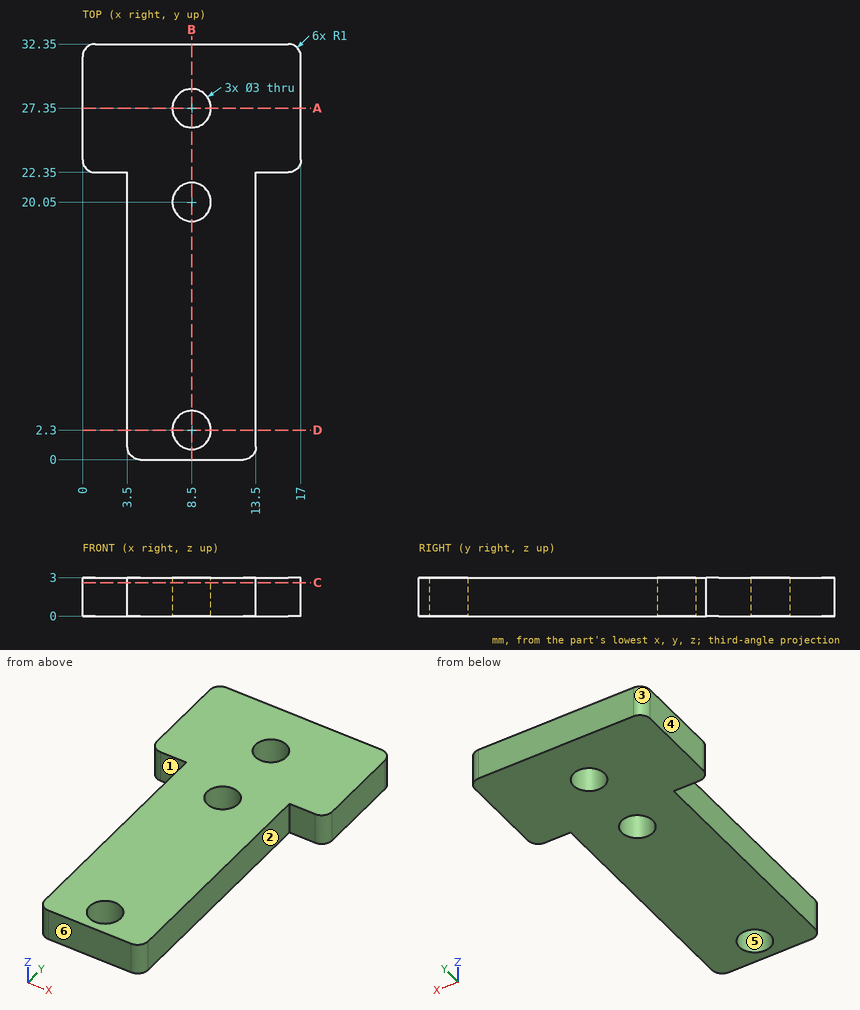
For this review, use the dimensioned drawing (mm, ordinates from the lowest corner) and the shaded views. A direction names the side the tool comes from. Give positions to 0.01 mm unless a question says otherwise; leave off trailing zeros. Order: outer loops, then holes, each group sorted by start corner. A loop starts at its lowest first (then second) coordinate and runs counter-clockwise, first axis right, second up. Notation, with made-up numbers: M -4.75,-21.75 L 45.25,-21.75 A26 cw 45.25,17.25 Z; hole C 85,10.5 d11. An arc over 180 degrees is marked long. Use one line per item in the form item = value. Start each with the question number.
Item 1: We need section A-A on y = 27.35. Give the boundary of the cut face in (x, z).
Item 2: We need section D-D on y = 2.3. Give the boundary of the cut face in (x, z), plus the area to 3 significant figures.
Item 3: The part is to be moulded in two halves that separate along Y. For the marked faces 4, 5 and 6, say which applies: pulls with the +Y half, pulls with the -Y half, needs draft (parallel to the pull), parting line crosses it, or undercut.
Item 4: We need section B-B on x = 8.5. Give the boundary of the cut face in (y, z).
Item 5: To check wall thickness, follow line 1 along Y through (x, z) = (8.5, 1.3); line 2 along Y through (x, z) = (9, 2.8); line 3 along X through (y, z) = (13, 1.4). State the ranges of each line that lie inside material, in increasing order. Write a range as from..to.
Item 6: Insertion check: pin 1 Ø1 at (y, z) = (8, 2) entering from +X; pin 2 Ø1.2 at (x, z) = (15, 1) entering from -Y; pin 3 Ø0.9 at (y, z) = (7.5, 1.5) entering from -X. Each pin has a flat end and moves straight along its axis. Give the tip position at first contact, or say it passes through.
Item 7: We need section C-C on z = 2.6. Give the boundary of the cut face in (x, y).
Item 8: For the marked faces 1, 2 and 3, list the 3-axis set-ups (+Z, -Z, +X, -X, +Y, -Y) from which the entire face can be reached by the end or side of a thin tool; tool diameter is ignored.
Completed:
q1.outline = M 0,0 L 7,0 L 7,3 L 0,3 Z; M 10,0 L 17,0 L 17,3 L 10,3 Z
q2.outline = M 3.5,0 L 7,0 L 7,3 L 3.5,3 Z; M 10,0 L 13.5,0 L 13.5,3 L 10,3 Z
q2.area = 21.0 mm²
q3.face_4 = needs draft
q3.face_5 = undercut
q3.face_6 = pulls with the -Y half
q4.outline = M 0,0 L 0.8,0 L 0.8,3 L 0,3 Z; M 3.8,0 L 18.55,0 L 18.55,3 L 3.8,3 Z; M 21.55,0 L 25.85,0 L 25.85,3 L 21.55,3 Z; M 28.85,0 L 32.35,0 L 32.35,3 L 28.85,3 Z
q5.line_1 = 0..0.8, 3.8..18.55, 21.55..25.85, 28.85..32.35
q5.line_2 = 0..0.89, 3.71..18.64, 21.46..25.94, 28.76..32.35
q5.line_3 = 3.5..13.5
q6.pin_1 = 13.5
q6.pin_2 = 22.35
q6.pin_3 = 3.5
q7.outline = M 0,23.35 A1 ccw 1,22.35 L 3.5,22.35 L 3.5,1 A1 ccw 4.5,0 L 12.5,0 A1 ccw 13.5,1 L 13.5,22.35 L 16,22.35 A1 ccw 17,23.35 L 17,31.35 A1 ccw 16,32.35 L 1,32.35 A1 ccw 0,31.35 Z; hole C 8.5,2.3 d3; hole C 8.5,20.05 d3; hole C 8.5,27.35 d3
q8.face_1 = +Z, -Z, -X, -Y
q8.face_2 = +Z, -Z, +X, -Y
q8.face_3 = +Z, -Z, -X, +Y
